Autodesk Inventor part; units mm, degrees
ref_plane "YZ Plane" through (0, 0, 0) normal (1, 0, 0) x (0, 1, 0)
ref_plane "XZ Plane" through (0, 0, 0) normal (0, 1, 0) x (-1, 0, 0)
ref_plane "XY Plane" through (0, 0, 0) normal (0, 0, 1) x (1, 0, 0)
sketch "Эскиз1" plane through (0, 0, 0) normal (0, 0, 1) x (1, 0, 0)
  line L0 (0, 4.3013) -> (3.725, 2.1506)
  line L1 (3.725, 2.1506) -> (3.725, -2.1506)
  line L2 (3.725, -2.1506) -> (0, -4.3013)
  line L3 (0, -4.3013) -> (-3.725, -2.1506)
  line L4 (-3.725, -2.1506) -> (-3.725, 2.1506)
  line L5 (-3.725, 2.1506) -> (0, 4.3013)
  circle A0 centre (0, 0) radius 12.5 construction
  arc A1 (1.0318, 12.4573) -> (-1.0292, 12.4147) centre (0, 12.5) ccw
  arc A2 (-1.0292, 12.4147) -> (-3.069, 12.1174) centre (-2.0583, 12.3294) ccw construction
  arc A3 (-3.069, 12.1174) -> (-1.0292, 12.4147) centre (-2.0583, 12.3294) ccw
  arc A4 (-1.0292, 12.4147) -> (1.0318, 12.4573) centre (0, 12.5) ccw construction
  arc A5 (-3.069, 12.1174) -> (-5.0044, 11.4079) centre (-4.0587, 11.8227) ccw
  arc A6 (-5.0044, 11.4079) -> (-6.8372, 10.4643) centre (-5.9501, 10.993) ccw construction
  arc A7 (-6.8372, 10.4643) -> (-5.0044, 11.4079) centre (-5.9501, 10.993) ccw
  arc A8 (-5.0044, 11.4079) -> (-3.069, 12.1174) centre (-4.0587, 11.8227) ccw construction
  arc A9 (-6.8372, 10.4643) -> (-8.4374, 9.1648) centre (-7.6777, 9.8643) ccw
  arc A10 (-8.4374, 9.1648) -> (-9.8645, 7.6773) centre (-9.1971, 8.4654) ccw construction
  arc A11 (-9.8645, 7.6773) -> (-8.4374, 9.1648) centre (-9.1971, 8.4654) ccw
  arc A12 (-8.4374, 9.1648) -> (-6.8372, 10.4643) centre (-7.6777, 9.8643) ccw construction
  arc A13 (-9.8645, 7.6773) -> (-10.9561, 5.9286) centre (-10.4646, 6.8369) ccw
  arc A14 (-10.9561, 5.9286) -> (-11.8229, 4.0583) centre (-11.4475, 5.0204) ccw construction
  arc A15 (-11.8229, 4.0583) -> (-10.9561, 5.9286) centre (-11.4475, 5.0204) ccw
  arc A16 (-10.9561, 5.9286) -> (-9.8645, 7.6773) centre (-10.4646, 6.8369) ccw construction
  arc A17 (-11.8229, 4.0583) -> (-12.2874, 2.05) centre (-12.1175, 3.0686) ccw
  arc A18 (-12.2874, 2.05) -> (-12.5, -0.0004) centre (-12.4574, 1.0314) ccw construction
  arc A19 (-12.5, -0.0004) -> (-12.2874, 2.05) centre (-12.4574, 1.0314) ccw
  arc A20 (-12.2874, 2.05) -> (-11.8229, 4.0583) centre (-12.1175, 3.0686) ccw construction
  arc A21 (-12.5, -0.0004) -> (-12.2873, -2.0508) centre (-12.4573, -1.0322) ccw
  arc A22 (-12.2873, -2.0508) -> (-11.8226, -4.0592) centre (-12.1173, -3.0694) ccw construction
  arc A23 (-11.8226, -4.0592) -> (-12.2873, -2.0508) centre (-12.1173, -3.0694) ccw
  arc A24 (-12.2873, -2.0508) -> (-12.5, -0.0004) centre (-12.4573, -1.0322) ccw construction
  arc A25 (-11.8226, -4.0592) -> (-10.9556, -5.9294) centre (-11.4472, -5.0212) ccw
  arc A26 (-10.9556, -5.9294) -> (-9.864, -7.678) centre (-10.4641, -6.8376) ccw construction
  arc A27 (-9.864, -7.678) -> (-10.9556, -5.9294) centre (-10.4641, -6.8376) ccw
  arc A28 (-10.9556, -5.9294) -> (-11.8226, -4.0592) centre (-11.4472, -5.0212) ccw construction
  arc A29 (-9.864, -7.678) -> (-8.4368, -9.1654) centre (-9.1965, -8.466) ccw
  arc A30 (-8.4368, -9.1654) -> (-6.8365, -10.4648) centre (-7.677, -9.8648) ccw construction
  arc A31 (-6.8365, -10.4648) -> (-8.4368, -9.1654) centre (-7.677, -9.8648) ccw
  arc A32 (-8.4368, -9.1654) -> (-9.864, -7.678) centre (-9.1965, -8.466) ccw construction
  arc A33 (-6.8365, -10.4648) -> (-5.0036, -11.4082) centre (-5.9493, -10.9934) ccw
  arc A34 (-5.0036, -11.4082) -> (-3.0681, -12.1176) centre (-4.0579, -11.823) ccw construction
  arc A35 (-3.0681, -12.1176) -> (-5.0036, -11.4082) centre (-4.0579, -11.823) ccw
  arc A36 (-5.0036, -11.4082) -> (-6.8365, -10.4648) centre (-5.9493, -10.9934) ccw construction
  arc A37 (-3.0681, -12.1176) -> (-1.0283, -12.4148) centre (-2.0574, -12.3295) ccw
  arc A38 (-1.0283, -12.4148) -> (1.0327, -12.4573) centre (0.0009, -12.5) ccw construction
  arc A39 (1.0327, -12.4573) -> (-1.0283, -12.4148) centre (0.0009, -12.5) ccw
  arc A40 (-1.0283, -12.4148) -> (-3.0681, -12.1176) centre (-2.0574, -12.3295) ccw construction
  arc A41 (1.0327, -12.4573) -> (3.0585, -12.076) centre (2.0574, -12.3295) ccw
  arc A42 (3.0585, -12.076) -> (5.0216, -11.447) centre (4.0596, -11.8224) ccw construction
  arc A43 (5.0216, -11.447) -> (3.0585, -12.076) centre (4.0596, -11.8224) ccw
  arc A44 (3.0585, -12.076) -> (1.0327, -12.4573) centre (2.0574, -12.3295) ccw construction
  arc A45 (5.0216, -11.447) -> (6.8138, -10.4286) centre (5.9493, -10.9934) ccw
  arc A46 (6.8138, -10.4286) -> (8.4663, -9.1962) centre (7.6784, -9.8637) ccw construction
  arc A47 (8.4663, -9.1962) -> (6.8138, -10.4286) centre (7.6784, -9.8637) ccw
  arc A48 (6.8138, -10.4286) -> (5.0216, -11.447) centre (5.9493, -10.9934) ccw construction
  arc A49 (8.4663, -9.1962) -> (9.8308, -7.6511) centre (9.1965, -8.466) ccw
  arc A50 (9.8308, -7.6511) -> (10.9936, -5.949) centre (10.4651, -6.8361) ccw construction
  arc A51 (10.9936, -5.949) -> (9.8308, -7.6511) centre (10.4651, -6.8361) ccw
  arc A52 (9.8308, -7.6511) -> (8.4663, -9.1962) centre (9.1965, -8.466) ccw construction
  arc A53 (10.9936, -5.949) -> (11.7824, -4.0445) centre (11.4472, -5.0212) ccw
  arc A54 (11.7824, -4.0445) -> (12.3296, -2.057) centre (12.1177, -3.0677) ccw construction
  arc A55 (12.3296, -2.057) -> (11.7824, -4.0445) centre (12.1177, -3.0677) ccw
  arc A56 (11.7824, -4.0445) -> (10.9936, -5.949) centre (11.4472, -5.0212) ccw construction
  arc A57 (12.3296, -2.057) -> (12.4573, 0.0004) centre (12.4573, -1.0322) ccw
  arc A58 (12.4573, 0.0004) -> (12.3294, 2.0579) centre (12.4572, 1.0331) ccw construction
  arc A59 (12.3294, 2.0579) -> (12.4573, 0.0004) centre (12.4572, 1.0331) ccw
  arc A60 (12.4573, 0.0004) -> (12.3296, -2.057) centre (12.4573, -1.0322) ccw construction
  arc A61 (12.3294, 2.0579) -> (11.7822, 4.0453) centre (12.1175, 3.0686) ccw
  arc A62 (11.7822, 4.0453) -> (10.9932, 5.9497) centre (11.4468, 5.022) ccw construction
  arc A63 (10.9932, 5.9497) -> (11.7822, 4.0453) centre (11.4468, 5.022) ccw
  arc A64 (11.7822, 4.0453) -> (12.3294, 2.0579) centre (12.1175, 3.0686) ccw construction
  arc A65 (10.9932, 5.9497) -> (9.8303, 7.6518) centre (10.4646, 6.8369) ccw
  arc A66 (9.8303, 7.6518) -> (8.4657, 9.1968) centre (9.1959, 8.4667) ccw construction
  arc A67 (8.4657, 9.1968) -> (9.8303, 7.6518) centre (9.1959, 8.4667) ccw
  arc A68 (9.8303, 7.6518) -> (10.9932, 5.9497) centre (10.4646, 6.8369) ccw construction
  arc A69 (8.4657, 9.1968) -> (6.8131, 10.429) centre (7.6777, 9.8643) ccw
  arc A70 (6.8131, 10.429) -> (5.0208, 11.4473) centre (5.9486, 10.9938) ccw construction
  arc A71 (5.0208, 11.4473) -> (6.8131, 10.429) centre (5.9486, 10.9938) ccw
  arc A72 (6.8131, 10.429) -> (8.4657, 9.1968) centre (7.6777, 9.8643) ccw construction
  arc A73 (5.0208, 11.4473) -> (3.0577, 12.0762) centre (4.0587, 11.8227) ccw
  arc A74 (3.0577, 12.0762) -> (1.0318, 12.4573) centre (2.0566, 12.3297) ccw construction
  arc A75 (1.0318, 12.4573) -> (3.0577, 12.0762) centre (2.0566, 12.3297) ccw
  arc A76 (3.0577, 12.0762) -> (5.0208, 11.4473) centre (4.0587, 11.8227) ccw construction
  circle A77 centre (0, 0) radius 2.1
  point P0 (-1.0318, 12.4573)
  point P1 (-5.0208, 11.4473)
  point P2 (-8.4657, 9.1968)
  point P3 (-10.9932, 5.9497)
  point P4 (-12.3294, 2.0579)
  point P5 (-12.3296, -2.057)
  point P6 (-10.9936, -5.949)
  point P7 (-8.4663, -9.1962)
  point P8 (-5.0216, -11.447)
  point P9 (-1.0327, -12.4573)
  point P10 (3.0681, -12.1176)
  point P11 (6.8365, -10.4648)
  point P12 (9.864, -7.678)
  point P13 (11.8226, -4.0592)
  point P14 (12.5, -0.0004)
  point P15 (11.8229, 4.0583)
  point P16 (9.8645, 7.6773)
  point P17 (6.8372, 10.4643)
  point P18 (3.069, 12.1174)
  point P19 (5.0208, 11.4473)
  point P20 (1.0318, 12.4573)
  point P21 (-3.069, 12.1174)
  point P22 (-9.8645, 7.6773)
  point P23 (-12.5, -0.0004)
  point P24 (-11.8226, -4.0592)
  point P25 (-9.864, -7.678)
  point P26 (-6.8365, -10.4648)
  point P27 (-3.0681, -12.1176)
  point P28 (1.0327, -12.4573)
  point P29 (5.0216, -11.447)
  point P30 (8.4663, -9.1962)
  point P31 (12.3296, -2.057)
  point P32 (12.3294, 2.0579)
  point P33 (10.9932, 5.9497)
  point P34 (8.4657, 9.1968)
  dimension "d0" = 7.45
  dimension "d1" = 25
  dimension "d6" = 360
  dimension "d8" = 4.2
extrude "Выдавливание1" add sketch "Эскиз1" along normal blind 4 contours A75 A73 A71 A69 A67 A65 A63 A61 A59 A57 A55 A53 A51 A49 A47 A45 A43 A41 A39 A37 A35 A33 A31 A29 A27 A25 A23 A21 A19 A17 A15 A13 A11 A9 A7 A5 A3 A1
extrude "Выдавливание2" add sketch "Эскиз1" along normal blind 1 contours L0 L1 L2 L3 L4 L5
properties part number "X_belt3"
Read the model definition and answer for the solid it produces. Units are mm, in the model's axes. A direction names the side the tool comes from. Coordinates: 2 decimals unless noted, no trailing zeros. Loops run counter-clockwise (first coordinate to the right, second up) from the corner with the lowest first, then second, coordinate; pieces in that order, holes last.
Q1. Which of the six approach directions +Z, -Z, +X, -X, +Y, -Y give full straight-line access (tool end or side, diameter ignored) to faces 1 (the face through (1.89, -3.21, 2.48)), 2 (the face through (-3.723, -10.846, 1.972))?
Q2. The part is cut by section B-B on x = -4.5. Write down the section's boundary in (y, z).
Q3. The mould has two halves that part along X. Classify faces 3 (the face through (-0.04, 13.53, 1.97)), 4 (the face through (3, -3, 4)): +X half, -X half, draft (parallel to the pull), parting line (faces both ways), or undercut.
Q4. Each of these flat-tipped pins is pushed along its axis until it touches: pin 1 Ø1.5 at (y, z) = (0, 2.5) entering from +X; pin 2 Ø4 at (x, y) = (0, 0) entering from -Z; pin 3 Ø1.5 at (y, z) = (-6.5, 1) entering from -X. Where does it stop, or does it pass through?
Q5. The part is cut by section A-A on y = -3.5. Write down the section's boundary in (x, z).
Q6. The part is cut by section C-C on y = 7. Write down the section's boundary in (x, z), and give its area (3 significant figures).
Q7. Consider probe 1 along X at (y, z) = (-1, 3.65) (3 decimals); probe 2 along Y at (x, z) = (0, 0.7); probe 3 along Y at (x, z) = (-11.25, 3.15). Determine where each line is inside the solid, lowest interval first.
Results below:
1. face 1: +Z
1. face 2: +Z, -Z
2. outline: (-10.89, 0) - (12.76, 0) - (12.76, 4) - (-10.89, 4) - close
3. face 3: undercut
3. face 4: draft
4. pin 1: stops at x = 13.45
4. pin 2: passes through
4. pin 3: stops at x = -12.18
5. outline: (-11.18, 0) - (11.18, 0) - (11.18, 4) - (1.39, 4) - (1.39, 1) - (-1.39, 1) - (-1.39, 4) - (-11.18, 4) - close
6. outline: (-11.48, 0) - (11.48, 0) - (11.48, 4) - (-11.48, 4) - close
6. area: 91.9 mm2
7. probe 1: x = -13.489 to -3.725, 3.725 to 13.49
7. probe 2: y = -11.47 to -2.1, 2.1 to 13.53
7. probe 3: y = -6.03 to -3.63, -2.51 to 4.01, 6.17 to 7.51
